```python
from build123d import *

# Parameters (mm, degrees)
SKETCH1_W               = 45
SKETCH1_H               = 38.8
BOSS_EXTRUDE1_DEPTH     = 0.79375
CUT_EXTRUDE1_DEPTH      = 30.751137058
CUT_EXTRUDE1_DEPTH_BACK = 30.751137058
SKETCH2_R               = 1.65
CHAMFER1_SIZE           = 2.8
FILLET1_R               = 2


with BuildPart() as part:
    # Sketch1 → Boss-Extrude1 (new, symmetric)
    with BuildSketch(Plane(origin=(0, 0, 0), x_dir=(1, 0, 0), z_dir=(0, 1, 0))):
        Rectangle(SKETCH1_W, SKETCH1_H)
    extrude(amount=BOSS_EXTRUDE1_DEPTH, both=True)

    # Sketch2 → Cut-Extrude1 (cut, two sides: drawn at the far end of the back side and taken through both)
    with BuildSketch(Plane(origin=(0, 0.79375, 0), x_dir=(1, 0, 0), z_dir=(0, 1, 0)).offset(-CUT_EXTRUDE1_DEPTH_BACK)):
        with Locations(Location((-17.5, 16.7, 0), (0, 0, 270))):
            Circle(SKETCH2_R)
        with Locations(Location((17.5, 16.7, 0), (0, 0, 270))):
            Circle(SKETCH2_R)
        with Locations(Location((17.5, -16.7, 0), (0, 0, 270))):
            Circle(SKETCH2_R)
        with Locations(Location((-17.5, -16.7, 0), (0, 0, 270))):
            Circle(SKETCH2_R)
    extrude(amount=CUT_EXTRUDE1_DEPTH + CUT_EXTRUDE1_DEPTH_BACK, mode=Mode.SUBTRACT)

    # Chamfer1
    chamfer1_edges = [part.edges().sort_by_distance(p)[0] for p in [
        (22.5, 0, 19.4),
        (-22.5, 0, 19.4),
        (-22.5, 0, -19.4),
        (22.5, 0, -19.4),
    ]]
    chamfer(chamfer1_edges, length=CHAMFER1_SIZE)

    # Fillet1
    fillet1_edges = [part.edges().sort_by_distance(p)[0] for p in [
        (19.7, 0, 19.4),
        (-19.7, 0, 19.4),
        (-22.5, 0, -16.6),
        (-22.5, 0, 16.6),
        (19.7, 0, -19.4),
        (-19.7, 0, -19.4),
        (22.5, 0, 16.6),
        (22.5, 0, -16.6),
    ]]
    fillet(fillet1_edges, radius=FILLET1_R)


solid = part.part
```
Can you work these out from the model? Positions are in its coordinate system, mm. Give positions to 0.01 mm unless a question says otherwise; leave off trailing zeros. Loops run counter-clockwise (first coordinate to the right, second up) from the corner with the lowest first, then second, coordinate; pieces in that order, holes last. Notation, with made-up numbers: M 43.25,19.5 L 81.25,19.5 A25 cw 81.25,57.5 Z; hole C -3.75,80.5 d6. An arc over 180 degrees is marked long. Use one line per item in the form item = value. Start each with the question number.
(1) Thinking about a two-plate mould opening in Z: for faces 1 (the cylindrical face through (17.996, -0.011, 18.274)), 2 (the cylindrical face through (22.344, -0.011, -16.547)), 3 (the cylindrical face through (22.344, 0.011, 16.547)), which applies, released by +Z, released by -Z, zero draft, split by the parting line, or undercut?
(2) I'm going to push a flat-ended pin straight in: P1, Ø2.5, axis at x = 17.5, z = -16.7, coming from the +Y side. Where does the tip first touch, or does it pass through?
(3) I want a section at A-A, the plane x = 17.5. Write out the boundary of the cut face in (y, z), and give its area (3 significant figures).
(4) Please list where these lines run through material, in increasing order: line 1 (Z direction, x = -17.5, y = -0.05); line 2 (X direction, y = 0.2, z = 16.7); line 3 (X direction, y = 0.4, z = 16.5).
(5) I want a section at C-C, the plane z = 16.7. Write out the boundary of the cut face in (x, y), and give its area (3 significant figures).
(6) I want a section at B-B, the plane y = 0.3. Write out the boundary of the cut face in (x, z), and give its area (3 significant figures).
Worked out:
q1.face_1 = undercut
q1.face_2 = released by -Z
q1.face_3 = released by +Z
q2.P1 = through
q3.outline = M -0.79,-19.4 L 0.79,-19.4 L 0.79,-18.35 L -0.79,-18.35 Z; M -0.79,-15.05 L 0.79,-15.05 L 0.79,15.05 L -0.79,15.05 Z; M -0.79,18.35 L 0.79,18.35 L 0.79,19.4 L -0.79,19.4 Z
q3.area = 51.1 mm²
q4.line_1 = -19.4 to -18.35, -15.05 to 15.05, 18.35 to 19.4
q4.line_2 = -22.27 to -19.15, -15.85 to 15.85, 19.15 to 22.27
q4.line_3 = -22.36 to -19.14, -15.86 to 15.86, 19.14 to 22.36
q5.outline = M -22.27,-0.79 L -19.15,-0.79 L -19.15,0.79 L -22.27,0.79 Z; M -15.85,-0.79 L 15.85,-0.79 L 15.85,0.79 L -15.85,0.79 Z; M 19.15,-0.79 L 22.27,-0.79 L 22.27,0.79 L 19.15,0.79 Z
q5.area = 60.2 mm²
q6.outline = M -22.5,-15.77 A2 ccw -21.91,-17.19 L -20.29,-18.81 A2 ccw -18.87,-19.4 L 18.87,-19.4 A2 ccw 20.29,-18.81 L 21.91,-17.19 A2 ccw 22.5,-15.77 L 22.5,15.77 A2 ccw 21.91,17.19 L 20.29,18.81 A2 ccw 18.87,19.4 L -18.87,19.4 A2 ccw -20.29,18.81 L -21.91,17.19 A2 ccw -22.5,15.77 Z; hole C -17.5,-16.7 d3.3; hole C -17.5,16.7 d3.3; hole C 17.5,-16.7 d3.3; hole C 17.5,16.7 d3.3
q6.area = 1,700 mm²
